```python
from build123d import *

# Parameters (mm, degrees)
SKETCH_1_W      = 28
SKETCH_1_H      = 15.2
SKETCH_1_R      = 1.5
EXTRUDE_1_DEPTH = 2
SKETCH_2_W      = 5
SKETCH_2_H      = 5
EXTRUDE_2_DEPTH = 2
SKETCH_3_R      = 2
EXTRUDE_3_DEPTH = 2


with BuildPart() as part:
    # 草图1 → 凸台-拉伸1 (new body)
    with BuildSketch(Plane(origin=(0, 0, 0), x_dir=(1, 0, 0), z_dir=(0, 1, 0))):
        Rectangle(SKETCH_1_W, SKETCH_1_H)
        with Locations(Location((10.5, 0, 0), (0, 0, 270))):
            Circle(SKETCH_1_R, mode=Mode.SUBTRACT)
        with Locations(Location((-10.5, 0, 0), (0, 0, 270))):
            Circle(SKETCH_1_R, mode=Mode.SUBTRACT)
    extrude(amount=EXTRUDE_1_DEPTH)

    # 草图2 → 凸台-拉伸2 (add)
    with BuildSketch(Plane(origin=(0, 2, 0), x_dir=(1, 0, 0), z_dir=(0, 1, 0))):
        with Locations((4.5, 0)):
            Rectangle(SKETCH_2_W, SKETCH_2_H)
        with Locations((-4.5, 0)):
            Rectangle(SKETCH_2_W, SKETCH_2_H)
    extrude(amount=EXTRUDE_2_DEPTH)

    # 草图3 → 凸台-拉伸3 (add)
    with BuildSketch(Plane(origin=(0, 4, 0), x_dir=(1, 0, 0), z_dir=(0, 1, 0))):
        with Locations(Location((4.5, 0, 0), (0, 0, 270))):
            Circle(SKETCH_3_R)
        with Locations(Location((-4.5, 0, 0), (0, 0, 90))):
            Circle(SKETCH_3_R)
    extrude(amount=EXTRUDE_3_DEPTH)


solid = part.part
```
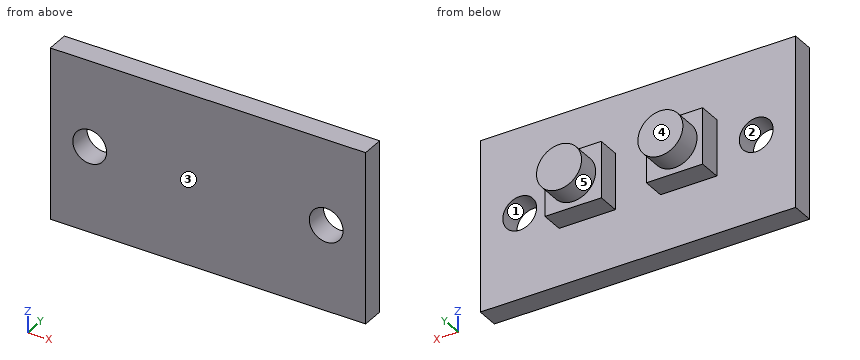
Can you work these out from the model? Positions are in its coordinate system, mm. Face numbers are marked on the shaded views. A direction names the side the tool comes from. Round coordinates to 2 decimals unless told otherwise and drop trailing zeros. Loops run counter-clockwise (first coordinate to the right, second up) from the corner with the lowest first, then second, coordinate; pieces in that order, holes last. Notation, with made-up numbers: M 53.5,49.5 L 86.5,49.5 A25 cw 86.5,70.5 Z; hole C 15,63 d10. An arc over 180 degrees is marked long. Answer as a JSON object with one key per item and string values. Group by question number.
Q1. Will these pins go through, and if not, where does the flat tip stop? pin 1 (1.6 mm diameter, centred on y = 3, z = 1, fed in from -X); pin 2 (2 mm diameter, centred on x = 4, y = 3.5, fed in from +Z); pin 3 (3.5 mm diameter, centred on x = -10.5, z = 0, fed in from +Y).
Q2. Imagine slicing it at C-C, the plane y = 0.6. Please give me the cut outline in (x, z), then the cut area to 3 significant figures.
Q3. Please list where these lines run through material, in increasing order: L1, parallel to X at y = 1.35, z = 0; L2, parallel to Z at x = 6.25, y = 3.9; L3, parallel to Z at x = 10.25, y = 0.65.
Q4. Imagine slicing it at A-A, the plane x = -10.5. Please give me the cut outline in (y, z), then the cut area to 3 significant figures.
Q5. On a 3-axis mill with a long thin cutter (end or side, diameter ignored), from which of +Z, -Z, +X, -X, +Y, -Y can I reach the whole of each face in a straight line? I mean the marked faces 4 and 5. Say none if no direction works.
Q6. Imagine slicing it at D-D, the plane x = 4.5. Please give me the cut outline in (y, z).
Q7. We'd pull the mould along X, two halves only. Please class the marked faces 1, 2 and 3: +X half, -X half, draft (parallel to the pull), parting line (faces both ways), or undercut.
Q8. Imagine slicing it at B-B, the plane y = 2.3. Please give me the cut outline in (x, z), then the cut area to 3 significant figures.
Findings:
{
 "1": {"pin 1": "stops at x = -7", "pin 2": "stops at z = 2.5", "pin 3": "stops at y = 2"},
 "2": {"outline": "M -14,-7.6 L 14,-7.6 L 14,7.6 L -14,7.6 Z; hole C -10.5,0 d3; hole C 10.5,0 d3", "area": "411 mm2"},
 "3": {"L1": "x = -14 to -12, -9 to 9, 12 to 14", "L2": "z = -2.5 to 2.5", "L3": "z = -7.6 to -1.48, 1.48 to 7.6"},
 "4": {"outline": "M 0,-7.6 L 2,-7.6 L 2,-1.5 L 0,-1.5 Z; M 0,1.5 L 2,1.5 L 2,7.6 L 0,7.6 Z", "area": "24.4 mm2"},
 "5": {"face 4": "+Z, -Z, +X, -X, +Y", "face 5": "+Y"},
 "6": {"outline": "M 0,-7.6 L 2,-7.6 L 2,-2.5 L 4,-2.5 L 4,-2 L 6,-2 L 6,2 L 4,2 L 4,2.5 L 2,2.5 L 2,7.6 L 0,7.6 Z"},
 "7": {"face 1": "undercut", "face 2": "undercut", "face 3": "draft"},
 "8": {"outline": "M -7,-2.5 L -2,-2.5 L -2,2.5 L -7,2.5 Z; M 2,-2.5 L 7,-2.5 L 7,2.5 L 2,2.5 Z", "area": "50.0 mm2"}
}
